Design review of the part built by this model. Coordinates are the model's own, in mm. Face numbers are marked on the shaded views. Coordinates: 2 decimals unless noted, no trailing zeros. Loops run counter-clockwise (first coordinate to the right, second up) from the corner with the lowest first, then second, coordinate; pieces in that order, holes last. Notation, with made-up numbers: (2.25, 10) -> (61.25, 10) arc R27 cw to (61.25, 41) -> close; hole circle Ø9 at (67, -40). An arc over 180 degrees is marked (long way). Answer as a JSON object with one key per item and string values.
```python
from build123d import *

# Parameters (mm, degrees)
SKETCH1_R               = 4.35
SKETCH1_R_2             = 2.8
BOSS_EXTRUDE1_DEPTH     = 5.45
SKETCH2_R               = 4.35
BOSS_EXTRUDE2_DEPTH     = 2.3
CUT_EXTRUDE2_REACH      = 22.657
SKETCH3_R               = 0.75
LPATTERN1_COUNT         = 4
LPATTERN1_PITCH         = 3
MIRROR1_COPY_1_REACH    = 22.657
MIRROR1_COPY_1_SKETCH_R = 0.75
MIRROR1_COPY_2_REACH    = 22.657
MIRROR1_COPY_2_SKETCH_R = 0.75
MIRROR1_COPY_3_REACH    = 22.657
MIRROR1_COPY_3_SKETCH_R = 0.75
SKETCH5_R               = 2.8
SKETCH5_R_2             = 1.5
BOSS_EXTRUDE3_DEPTH     = 2


with BuildPart() as part:
    # Sketch1 → Boss-Extrude1 (new body)
    with BuildSketch(Plane(origin=(0, 0, 0), x_dir=(1, 0, 0), z_dir=(0, 1, 0))):
        with Locations(Location((0, 0, 0), (0, 0, 270))):
            Circle(SKETCH1_R)
        with Locations(Location((0, 0, 0), (0, 0, 270))):
            Circle(SKETCH1_R_2, mode=Mode.SUBTRACT)
    extrude(amount=BOSS_EXTRUDE1_DEPTH)

    # Sketch2 → Boss-Extrude2 (add)
    with BuildSketch(Plane(origin=(0, 0, 0), x_dir=(1, 0, 0), z_dir=(0, 1, 0))):
        with BuildLine():
            ThreePointArc((2.98678731, 16.28125), (0, 19), (-2.98678731, 16.28125))
            Line((-2.98678731, 16.28125), (-4.108122187, 4.373023221))
            ThreePointArc((-4.108122187, 4.373023221), (-6, 0), (-4.108122187, -4.373023221))
            Line((-4.108122187, -4.373023221), (-2.98678731, -16.28125))
            ThreePointArc((-2.98678731, -16.28125), (0, -19), (2.98678731, -16.28125))
            Line((2.98678731, -16.28125), (4.108122187, -4.373023221))
            ThreePointArc((4.108122187, -4.373023221), (6, 0), (4.108122187, 4.373023221))
            Line((4.108122187, 4.373023221), (2.98678731, 16.28125))
        make_face()
        with Locations(Location((0, 0, 0), (0, 0, 270))):
            Circle(SKETCH2_R, mode=Mode.SUBTRACT)
    extrude(amount=BOSS_EXTRUDE2_DEPTH)

    # Sketch3 → Cut-Extrude2 (cut, up to next)
    with BuildSketch(Plane(origin=(0, 0, 0), x_dir=(1, 0, 0), z_dir=(0, 1, 0)), mode=Mode.PRIVATE) as cut_extrude2_sk1:
        with Locations(Location((0, 7, 0), (0, 0, 270))):
            Circle(SKETCH3_R)
    cut_extrude2_tool1 = extrude(cut_extrude2_sk1.sketch, amount=CUT_EXTRUDE2_REACH, mode=Mode.PRIVATE) & part.part
    cut_extrude2 = cut_extrude2_tool1.solids().sort_by_distance((0, 0, -7))[0]
    add(cut_extrude2, mode=Mode.SUBTRACT)

    # LPattern1: Cut-Extrude2 ×4
    with Locations(*[(0, 0, -i * LPATTERN1_PITCH) for i in range(1, LPATTERN1_COUNT)]):
        add(cut_extrude2, mode=Mode.SUBTRACT)

    # Mirror1: Cut-Extrude2 across plane
    add(cut_extrude2.mirror(Plane.XY), mode=Mode.SUBTRACT)

    # Mirror1 copy 1 sketch → Mirror1 copy 1 (cut, up to next)
    with BuildSketch(Plane(origin=(0, 0, 3), x_dir=(1, 0, 0), z_dir=(0, 1, 0)), mode=Mode.PRIVATE) as mirror1_copy_1_sk1:
        with Locations((0, -7)):
            Circle(MIRROR1_COPY_1_SKETCH_R)
    mirror1_copy_1_tool1 = extrude(mirror1_copy_1_sk1.sketch, amount=MIRROR1_COPY_1_REACH, mode=Mode.PRIVATE) & part.part
    add(mirror1_copy_1_tool1.solids().sort_by_distance((0, 0, 10))[0], mode=Mode.SUBTRACT)

    # Mirror1 copy 2 sketch → Mirror1 copy 2 (cut, up to next)
    with BuildSketch(Plane(origin=(0, 0, 6), x_dir=(1, 0, 0), z_dir=(0, 1, 0)), mode=Mode.PRIVATE) as mirror1_copy_2_sk1:
        with Locations((0, -7)):
            Circle(MIRROR1_COPY_2_SKETCH_R)
    mirror1_copy_2_tool1 = extrude(mirror1_copy_2_sk1.sketch, amount=MIRROR1_COPY_2_REACH, mode=Mode.PRIVATE) & part.part
    add(mirror1_copy_2_tool1.solids().sort_by_distance((0, 0, 13))[0], mode=Mode.SUBTRACT)

    # Mirror1 copy 3 sketch → Mirror1 copy 3 (cut, up to next)
    with BuildSketch(Plane(origin=(0, 0, 9), x_dir=(1, 0, 0), z_dir=(0, 1, 0)), mode=Mode.PRIVATE) as mirror1_copy_3_sk1:
        with Locations((0, -7)):
            Circle(MIRROR1_COPY_3_SKETCH_R)
    mirror1_copy_3_tool1 = extrude(mirror1_copy_3_sk1.sketch, amount=MIRROR1_COPY_3_REACH, mode=Mode.PRIVATE) & part.part
    add(mirror1_copy_3_tool1.solids().sort_by_distance((0, 0, 16))[0], mode=Mode.SUBTRACT)

    # Sketch5 → Boss-Extrude3 (add)
    with BuildSketch(Plane(origin=(0, 0, 0), x_dir=(1, 0, 0), z_dir=(0, 1, 0))):
        with Locations(Location((0, 0, 0), (0, 0, 270))):
            Circle(SKETCH5_R)
        with Locations(Location((0, 0, 0), (0, 0, 270))):
            Circle(SKETCH5_R_2, mode=Mode.SUBTRACT)
    extrude(amount=BOSS_EXTRUDE3_DEPTH)


solid = part.part
```
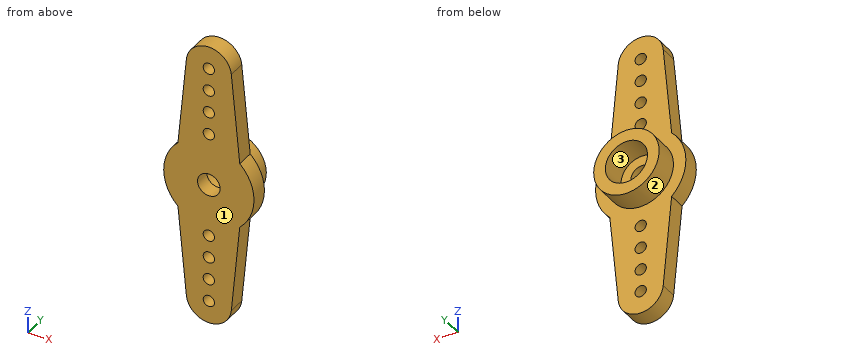
1) Clearance check with flat-ended pins moving along their axes: pin 1 Ø6 at (x, z) = (1, -0.5) entering from +Y; pin 2 Ø2.5 at (x, z) = (0, -10) entering from +Y. State where each tip first meets the part, or that it passes through.
Completed:
{"pin 1": "y = 5.45", "pin 2": "y = 2.3"}
2) Add section C-C, the plane z = -7. Give the boundary of the cut face in (x, y).
Completed:
{"outline": "(-3.86, 0) -> (-0.75, 0) -> (-0.75, 2.3) -> (-3.86, 2.3) -> close; (0.75, 0) -> (3.86, 0) -> (3.86, 2.3) -> (0.75, 2.3) -> close"}
3) Add section D-D, the plane x = -4.75. Give the boundary of the cut face in (y, z), and give its area (3 significant figures).
Completed:
{"outline": "(0, -3.67) -> (2.3, -3.67) -> (2.3, 3.67) -> (0, 3.67) -> close", "area": "16.9 mm²"}
4) The part is to be moulded in two halves that separate along Z. For the marked faces 1, 2 and 3, say which applies: pulls with the +Z half, pulls with the -Z half, needs draft (parallel to the pull), parting line crosses it, or undercut.
Completed:
{"face 1": "needs draft", "face 2": "parting line crosses it", "face 3": "undercut"}
5) Add section A-A, the plane z = 0. Give the boundary of the cut face in (x, y).
Completed:
{"outline": "(-6, 0) -> (-1.5, 0) -> (-1.5, 2) -> (-2.8, 2) -> (-2.8, 5.45) -> (-4.35, 5.45) -> (-4.35, 2.3) -> (-6, 2.3) -> close; (1.5, 0) -> (6, 0) -> (6, 2.3) -> (4.35, 2.3) -> (4.35, 5.45) -> (2.8, 5.45) -> (2.8, 2) -> (1.5, 2) -> close"}
6) Wall thickness on probe 1 along Y at (x, z) = (-4.75, -3); probe 2 along X at (y, z) = (1.25, 1); probe 3 along Z at (x, y) = (-0.75, 4.7): over which ranges is each line inside the solid? List them lowest first.
Completed:
{"probe 1": "0 to 2.3", "probe 2": "-5.92 to -1.12, 1.12 to 5.92", "probe 3": "-4.28 to -2.7, 2.7 to 4.28"}
7) Add section B-B, the plane y = 2.85. Give the boundary of the cut face in (x, z).
Completed:
{"outline": "circle Ø8.7 at (0, 0); hole circle Ø5.6 at (0, 0)"}
